Check sheet for the drawn part. Datum: minimum x, y, z corner. Units: mm. A direction names the side the tool comes from. Round coordinates to 2 decimals unless told otherwise and drop trailing zeros. Write each loop counter-clockwise with the first axis right and the second up, starting at its lowest first coordinate (ties: lowest second). Pieces come first, ordered by that corner, then holes. Notation, with made-up numbers: M -14,58 L -6,58 A17 cw -6,70 Z; hole C 61,-39 d9. An arc over 180 degrees is marked long. One line per item, written item: value. Start each with the question number.
Item 1: Section check C-C, the plane x = 12.5. Record the cut outline in (y, z).
Item 2: Section check A-A, the plane z = 7. Record the cut outline in (x, y).
Item 3: Draft check along Y on the marked faces 3, 4 and 5. Enter one of: +Y half, -Y half, draft (parallel to the pull), parting line (faces both ways), or undercut.
Item 4: Thickness scan on probe 1 along Y at (x, z) = (15, 58); probe 2 along Z at (x, y) = (47.5, 10) (1 decimal); probe 3 along X at (y, z) = (36.6, 33). Record the ranges inside material, lowest first. Write a range as from..to.
Item 5: Gauge pin test, flat ends, axial feed: pin 1 (5 mm diameter, centred on y = 46, z = 41.5, fed in from -X); pin 2 (3 mm diameter, centred on x = 9.31, z = 33, fed in from -Y); pin 3 (8 mm diameter, centred on x = 27, z = 46, fed in from +Y); pin 4 (11 mm diameter, centred on x = 8, y = 49, fed in from +Z). Record the tip position at first contact, or that the pin passes through.
Item 6: Section check D-D, the plane z = 32.5. Record the cut outline in (x, y).
Item 7: Tool access check on the marked faces 1 and 2. Record the directions out of +Z, -Z, +X, -X, +Y, -Y that give a thin tool (end or side, any length) a straight path to the whole face; none if there is none.
Item 8: Section check B-B, the plane y = 44. Record the cut outline in (x, z), then the cut area to 3 significant figures.
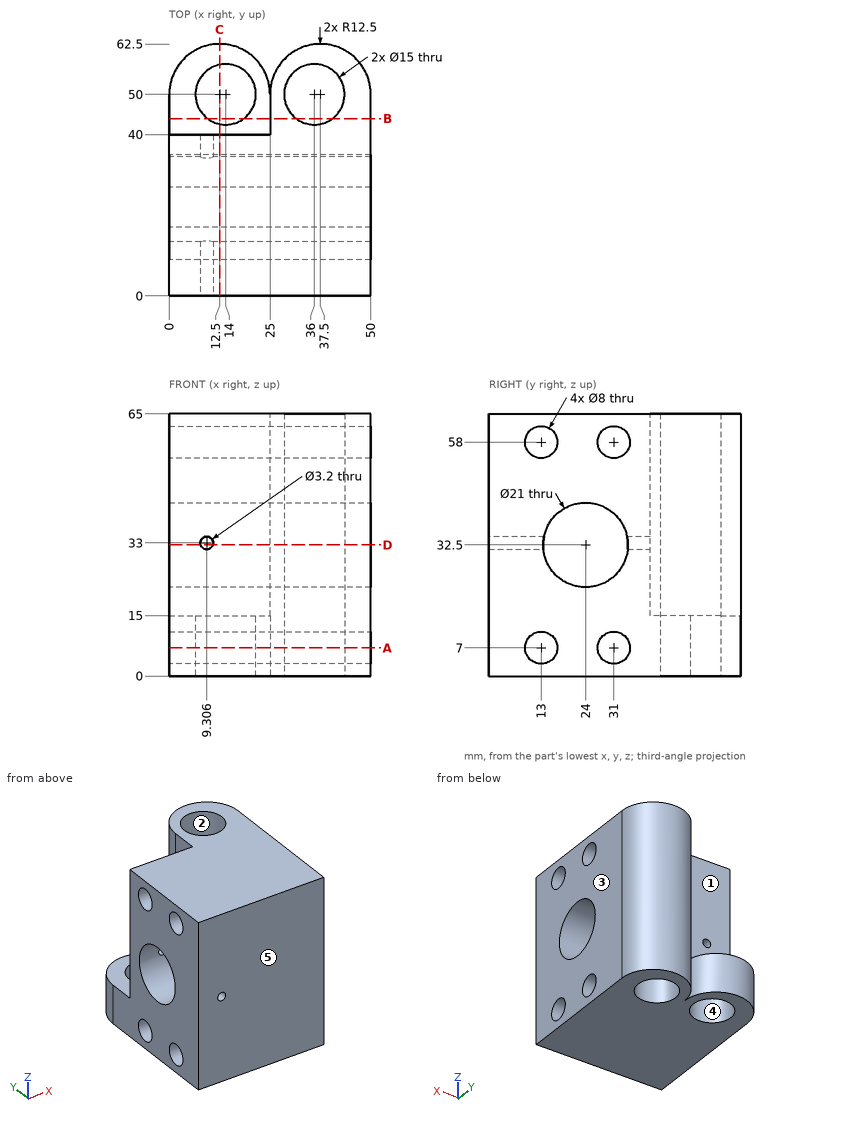
Response values:
1. outline: M 0,0 L 42.65,0 L 42.65,15 L 40,15 L 40,65 L 0,65 Z; M 57.35,0 L 62.5,0 L 62.5,15 L 57.35,15 Z; hole C 13,7 d8; hole C 13,58 d8; hole C 24,32.5 d21; hole C 31,7 d8; hole C 31,58 d8
2. outline: M 0,0 L 50,0 L 50,9 L 0,9 Z; M 0,17 L 50,17 L 50,27 L 0,27 Z; M 0,35 L 50,35 L 50,50 A12.5 ccw 25,50 A12.5 ccw 0,50 Z; hole C 14,50 d15; hole C 36,50 d15
3. face 3: draft
3. face 4: undercut
3. face 5: -Y half
4. probe 1: y = 0..9, 17..27, 35..40
4. probe 2: z = 0..4.4, 9.6..55.4, 60.6..65
4. probe 3: x = 0..7.71, 10.91..50
5. pin 1: stops at x = 25
5. pin 2: passes through
5. pin 3: stops at y = 60.68
5. pin 4: stops at z = 15
6. outline: M 0,0 L 7.79,0 L 7.79,13.5 L 0,13.5 Z; M 0,34.5 L 7.79,34.5 L 7.79,40 L 0,40 Z; M 10.83,0 L 50,0 L 50,13.5 L 10.83,13.5 Z; M 10.83,34.5 L 50,34.5 L 50,50 A12.5 ccw 25,50 L 25,40 L 10.83,40 Z; hole C 36,50 d15
7. face 1: +Z, -X, +Y
7. face 2: +Z, -Z
8. outline: M 0,0 L 9.5,0 L 9.5,15 L 0,15 Z; M 18.5,0 L 31.5,0 L 31.5,65 L 25,65 L 25,15 L 18.5,15 Z; M 40.5,0 L 50,0 L 50,65 L 40.5,65 Z
8. area: 1,280 mm2
